CAD build for the part. Positions are in the model's coordinates, mm. A direction names the side the tool comes from. Round coordinates to 2 decimals unless told otherwise and drop trailing zeros. Order: outer loops, then holes, each group sorted by start corner. A loop starts at its lowest first (then second) coordinate and runs counter-clockwise, first axis right, second up. Notation, with made-up numbers: M -18,50.25 L -14,50.25 A17 cw -14,75.25 Z; hole C 57,51 d5. An arc over 180 degrees is marked long. Answer as a JSON object with one key per item and string values.
Autodesk Inventor part; units mm, degrees
ref_plane "YZ Plane" through (0, 0, 0) normal (1, 0, 0) x (0, 1, 0)
ref_plane "XZ Plane" through (0, 0, 0) normal (0, 1, 0) x (-1, 0, 0)
ref_plane "XY Plane" through (0, 0, 0) normal (0, 0, 1) x (1, 0, 0)
sketch "Sketch1" plane through (0, 0, 0) normal (0, 0, 1) x (1, 0, 0)
  circle A0 centre (-15.5, -15.5) radius 1.2295 construction
  circle A1 centre (15.5, 15.5) radius 1.2295 construction
  circle A2 centre (15.5, -15.5) radius 1.2295 construction
  circle A3 centre (-15.5, 15.5) radius 1.2295 construction
  circle A4 centre (0, 0) radius 11 construction
  arc A5 (-16.5, 21) -> (-21, 16.5) centre (-16.5, 16.5) ccw construction
  line L0 (-21, 16.5) -> (-21, -16.5) construction
  arc A6 (-21, -16.5) -> (-16.5, -21) centre (-16.5, -16.5) ccw construction
  line L1 (-16.5, -21) -> (16.5, -21) construction
  arc A7 (16.5, -21) -> (21, -16.5) centre (16.5, -16.5) ccw construction
  line L2 (21, -16.5) -> (21, 16.5) construction
  arc A8 (21, 16.5) -> (16.5, 21) centre (16.5, 16.5) ccw construction
  line L3 (16.5, 21) -> (-16.5, 21) construction
  line L4 (16.5, 21) -> (-26.5, 21)
  line L5 (-31, 16.5) -> (-31, -16.5)
  line L6 (-26.5, -21) -> (16.5, -21)
  line L7 (21, -16.5) -> (21, 16.5)
  arc A9 (21, 16.5) -> (16.5, 21) centre (16.5, 16.5) ccw
  arc A10 (16.5, -21) -> (21, -16.5) centre (16.5, -16.5) ccw
  arc A11 (-31, -16.5) -> (-26.5, -21) centre (-26.5, -16.5) ccw
  arc A12 (-26.5, 21) -> (-31, 16.5) centre (-26.5, 16.5) ccw
  circle A13 centre (15.5, 15.5) radius 1.2295
  circle A14 centre (15.5, -15.5) radius 1.2295
  circle A15 centre (-15.5, -15.5) radius 1.2295
  circle A16 centre (-15.5, 15.5) radius 1.2295
  circle A17 centre (0, 0) radius 11 construction
  circle A18 centre (0, 0) radius 5 construction
  circle A19 centre (0, 0) radius 10 construction
  circle A20 centre (0, 0) radius 15 construction
  line L8 (-7, 3) -> (-7, -3) construction
  line L9 (-12, 3) -> (-12, -3) construction
  line L10 (-17, 3) -> (-17, -3) construction
  circle A21 centre (-7, 3) radius 1.5
  circle A22 centre (-7, -3) radius 1.5
  circle A23 centre (-12, 3) radius 1.5
  circle A24 centre (-12, -3) radius 1.5
  circle A25 centre (-17, 3) radius 1.5
  circle A26 centre (-17, -3) radius 1.5
  circle A27 centre (-25, 15.5) radius 1.5
  circle A28 centre (-25, -15.5) radius 1.5
  circle A29 centre (0, 0) radius 2.5
  point P0 (-7, 0)
  point P1 (-12, 0)
  point P2 (-17, 0)
  point P3 (-5, 0)
  point P4 (-10, 0)
  point P5 (-15, 0)
  point P6 (-10.5169, -3.2242)
  point P7 (-10.7969, -2.1042)
  point P8 (-10.7969, 2.1042)
  point P9 (-10.5169, 3.2242)
extrude "Extrusion1" add sketch "Sketch1" along normal blind 3.5
sketch "Sketch3" plane through (0, 0, 0) normal (0, 0, -1) x (-1, 0, 0)
  circle A0 centre (-15.5, 15.5) radius 1.2295
  circle A1 centre (15.5, 15.5) radius 1.2295
  circle A2 centre (15.5, -15.5) radius 1.2295
  circle A3 centre (-15.5, -15.5) radius 1.2295
  circle A4 centre (-15.5, 15.5) radius 4
  circle A5 centre (15.5, 15.5) radius 4
  circle A6 centre (15.5, -15.5) radius 4
  circle A7 centre (-15.5, -15.5) radius 4
  point P0 (0, 0)
  dimension "d37" = 8
  dimension "d38" = 8
  dimension "d39" = 8
  dimension "d40" = 8
extrude "Extrusion2" add sketch "Sketch3" along normal blind 4
equation "\"d38\" = d37"
equation "\"d39\" = d37"
equation "\"d40\" = d37"
equation "\"d6\" = d5"
equation "\"d7\" = d5"
properties part number "housing" material "PET Plastic"
Item 1: Saw through at A-A on z = -1.5. List the corners of the cut face in (x, y), and give its area (3 significant figures).
Worked answers:
{"outline": "C -15.5,-15.5 d8; C -15.5,15.5 d8; C 15.5,-15.5 d8; C 15.5,15.5 d8; hole C -15.5,-15.5 d2.46; hole C -15.5,15.5 d2.46; hole C 15.5,-15.5 d2.46; hole C 15.5,15.5 d2.46", "area": "182 mm2"}
Item 2: Two-plate mould, pull along Y, no slides. Class faces 1 (the cylindrical face through (-8.2, -2.1, 1.7)), 2 (the cylindrical face through (-29.717, 19.647, 1.726)), 3 (the flat face through (-31, 0, 2)): released by +Y, released by -Y, zero draft, split by the parting line, or undercut.
Worked answers:
{"face 1": "undercut", "face 2": "released by +Y", "face 3": "zero draft"}
Item 3: Saw through at C-C on y = 15.5. List the corners of the cut face in (x, z), and give its area (3 significant figures).
Worked answers:
{"outline": "M -31,0 L -26.5,0 L -26.5,3.5 L -31,3.5 Z; M -23.5,0 L -19.5,0 L -19.5,-4 L -16.73,-4 L -16.73,3.5 L -23.5,3.5 Z; M -14.27,-4 L -11.5,-4 L -11.5,0 L 11.5,0 L 11.5,-4 L 14.27,-4 L 14.27,3.5 L -14.27,3.5 Z; M 16.73,-4 L 19.5,-4 L 19.5,0 L 21,0 L 21,3.5 L 16.73,3.5 Z", "area": "199 mm2"}
Item 4: Wall check: line 1 along Y through (x, z) = (15.5, -3.1); line 2 along Y through (x, z) = (-17, 2.6); line 3 along Y through (x, z) = (16, 2.5). Give the ranges that are in metal, low to high. Write a range as [from, to].
Worked answers:
{"line 1": "y = [-19.5, -16.73], [-14.27, -11.5], [11.5, 14.27], [16.73, 19.5]", "line 2": "y = [-21, -4.5], [-1.5, 1.5], [4.5, 21]", "line 3": "y = [-21, -16.62], [-14.38, 14.38], [16.62, 21]"}
Item 5: Saw through at B-B on y = 0. List the corners of the cut face in (x, z).
Worked answers:
{"outline": "M -31,0 L -2.5,0 L -2.5,3.5 L -31,3.5 Z; M 2.5,0 L 21,0 L 21,3.5 L 2.5,3.5 Z"}
Item 6: Drop flat-ended pins along their axis: pin 1 Ø1.8 at (x, y) = (-12, -3) entering from -Z; pin 2 Ø12 at (x, y) = (3, 3.5) entering from -Z. Give the stop position or say it passes through.
Worked answers:
{"pin 1": "passes through", "pin 2": "stops at z = 0"}
Item 7: Saw through at D-D on x = 0. List the corners of the cut face in (y, z).
Worked answers:
{"outline": "M -21,0 L -2.5,0 L -2.5,3.5 L -21,3.5 Z; M 2.5,0 L 21,0 L 21,3.5 L 2.5,3.5 Z"}
Item 8: 3-axis set-ups, long thin cutter, end or side, ignore diameter. For faces 4 (the flat face through (-5, 0, 0)), 5 (the flat face through (-15, -17, -4)): which of +Z, -Z, +X, -X, +Y, -Y reach the whole face in a straight line?
Worked answers:
{"face 4": "-Z", "face 5": "-Z, +X, -X, +Y, -Y"}
